```python
from build123d import *

# Parameters (mm, degrees)
SKETCH_1131_R          = 3
EXTRUDE_1145_DEPTH     = 2
EXTRUDE_1198_DEPTH     = 30
SKETCH_1301_W          = 30
SKETCH_1301_H          = 5
CUT_EXTRUDE_1405_DEPTH = 10


with BuildPart() as part:
    # Sketch 1131 → Extrude 1145 (new body)
    with BuildSketch(Plane(origin=(0, 0, 0), x_dir=(1, 0, 0), z_dir=(0, 1, 0))):
        with BuildLine():
            Line((-90, 40), (90, 40))
            ThreePointArc((90, 40), (97.071067812, 37.071067812), (100, 30))
            Line((100, 30), (100, -40))
            Line((100, -40), (-100, -40))
            Line((-100, -40), (-100, 30))
            ThreePointArc((-100, 30), (-97.071067812, 37.071067812), (-90, 40))
        make_face()
        with Locations(Location((60, -25, 0), (0, 0, 270))):
            Circle(SKETCH_1131_R, mode=Mode.SUBTRACT)
        with Locations(Location((0, -25, 0), (0, 0, 270))):
            Circle(SKETCH_1131_R, mode=Mode.SUBTRACT)
        with Locations(Location((-60, -25, 0), (0, 0, 270))):
            Circle(SKETCH_1131_R, mode=Mode.SUBTRACT)
        with BuildLine():
            Line((49, 30), (71, 30))
            ThreePointArc((71, 30), (73.828427125, 28.828427125), (75, 26))
            Line((75, 26), (75, -1))
            ThreePointArc((75, -1), (73.828427125, -3.828427125), (71, -5))
            Line((71, -5), (49, -5))
            ThreePointArc((49, -5), (46.171572875, -3.828427125), (45, -1))
            Line((45, -1), (45, 26))
            ThreePointArc((45, 26), (46.171572875, 28.828427125), (49, 30))
        make_face(mode=Mode.SUBTRACT)
        with BuildLine():
            Line((-11, 30), (11, 30))
            ThreePointArc((11, 30), (13.828427125, 28.828427125), (15, 26))
            Line((15, 26), (15, -1))
            ThreePointArc((15, -1), (13.828427125, -3.828427125), (11, -5))
            Line((11, -5), (-11, -5))
            ThreePointArc((-11, -5), (-13.828427125, -3.828427125), (-15, -1))
            Line((-15, -1), (-15, 26))
            ThreePointArc((-15, 26), (-13.828427125, 28.828427125), (-11, 30))
        make_face(mode=Mode.SUBTRACT)
        with BuildLine():
            Line((-71, 30), (-49, 30))
            ThreePointArc((-49, 30), (-46.171572875, 28.828427125), (-45, 26))
            Line((-45, 26), (-45, -1))
            ThreePointArc((-45, -1), (-46.171572875, -3.828427125), (-49, -5))
            Line((-49, -5), (-71, -5))
            ThreePointArc((-71, -5), (-73.828427125, -3.828427125), (-75, -1))
            Line((-75, -1), (-75, 26))
            ThreePointArc((-75, 26), (-73.828427125, 28.828427125), (-71, 30))
        make_face(mode=Mode.SUBTRACT)
    extrude(amount=-EXTRUDE_1145_DEPTH)

    # Sketch 1191 → Extrude 1198 (add)
    with BuildSketch(Plane(origin=(0, 0, 0), x_dir=(1, 0, 0), z_dir=(0, 1, 0))):
        with BuildLine():
            Line((-90, 40), (90, 40))
            ThreePointArc((90, 40), (97.071067812, 37.071067812), (100, 30))
            Line((100, 30), (100, -40))
            Line((100, -40), (-100, -40))
            Line((-100, -40), (-100, 30))
            ThreePointArc((-100, 30), (-97.071067812, 37.071067812), (-90, 40))
        make_face()
        with BuildLine():
            Line((-90, 35), (90, 35))
            ThreePointArc((90, 35), (93.535533906, 33.535533906), (95, 30))
            Line((95, 30), (95, -35))
            Line((95, -35), (-95, -35))
            Line((-95, -35), (-95, 30))
            ThreePointArc((-95, 30), (-93.535533906, 33.535533906), (-90, 35))
        make_face(mode=Mode.SUBTRACT)
    extrude(amount=-EXTRUDE_1198_DEPTH)

    # Sketch 1301 → Cut-Extrude 1405 (cut)
    with BuildSketch(Plane(origin=(0, -30, 0), x_dir=(1, 0, 0), z_dir=(0, 1, 0))):
        with Locations((10, 37.5)):
            Rectangle(SKETCH_1301_W, SKETCH_1301_H)
    extrude(amount=CUT_EXTRUDE_1405_DEPTH, mode=Mode.SUBTRACT)


solid = part.part
```
Source: CAD feature listing. Evaluate the final solid. Frame: model axes, mm. A direction names the side the tool comes from. Coordinates: 2 decimals unless noted, no trailing zeros. Loops run counter-clockwise (first coordinate to the right, second up) from the corner with the lowest first, then second, coordinate; pieces in that order, holes last. Notation, with made-up numbers: M -27.75,-10 L -2.75,-10 A26 cw -2.75,29 Z; hole C 15.25,55 d9. An arc over 180 degrees is marked long. Put each result on its own line as item: value. Start each with the question number.
1) Cut plane B-B on z = -16. Return the cut outline in (x, y), then the cut area to 3 significant figures.
2) Cut plane A-A on x = 0. Return the cut outline in (y, z).
3) Reachability of faces 1 (the face through (10, -20, -38)), 2 (the face through (93, -16, -34)), 3 (the face through (-46.141, -0.986, 3.797)) from +Z, -Z, +X, -X, +Y, -Y: full face, straight path, thin tool, end or side. Return the list, or none.
4) Contact query for flat-ended pins moving along their axis: pin 1 Ø5.5 at (y, z) = (-23, -37) entering from -X; pin 2 Ø9.5 at (x, z) = (0, 25) entering from +Y. Output: stop coordinate, or through.
5) Pull-direction query (Z, two-part tool) for faces 4 (the face through (-13.797, -0.986, 3.859)), 5 (the face through (-97.15, -14.79, -36.99)), 6 (the face through (73.859, -0.986, 3.797)), 7 (the face through (100, -15, 5)); classes: pulls with the +Z half, pulls with the -Z half, needs draft (parallel to the pull), parting line crosses it, or undercut.
6) Cut plane D-D on y = -7.75. Return the cut outline in (x, z), then the cut area to 3 significant figures.
7) Ray query, L1, parallel to X at y = -1.5, z = 25; L2, parallel to X at y = -20.25, z = 9.5; L3, parallel to Z at x = 52, y = -20.75. Return the intervals inside material, ascending. Write a range as from..to.
8) Cut plane C-C on x = -53. Return the cut outline in (y, z).
The answers:
1. outline: M -100,-30 L -95,-30 L -95,-2 L -75,-2 L -75,0 L -100,0 Z; M -45,-2 L -15,-2 L -15,0 L -45,0 Z; M 15,-2 L 45,-2 L 45,0 L 15,0 Z; M 75,-2 L 95,-2 L 95,-30 L 100,-30 L 100,0 L 75,0 Z
1. area: 500 mm²
2. outline: M -30,35 L -2,35 L -2,28 L 0,28 L 0,40 L -30,40 Z; M -20,-40 L 0,-40 L 0,-30 L -2,-30 L -2,-35 L -20,-35 Z; M -2,5 L 0,5 L 0,22 L -2,22 Z
3. face 1: -Z, -Y
3. face 2: -Y
3. face 3: +Y, -Y
4. pin 1: stops at x = -99.05
4. pin 2: stops at y = 0
5. face 4: undercut
5. face 5: pulls with the -Z half
5. face 6: undercut
5. face 7: needs draft
6. outline: M -100,-30 A10 ccw -90,-40 L 90,-40 A10 ccw 100,-30 L 100,40 L -100,40 Z; hole M -95,-30 A5 ccw -90,-35 L 90,-35 A5 ccw 95,-30 L 95,35 L -95,35 Z
6. area: 2,670 mm²
7. L1: x = -100..-63, -57..-3, 3..57, 63..100
7. L2: x = -100..-95, 95..100
7. L3: z = -40..-35, 35..40
8. outline: M -30,-40 L 0,-40 L 0,-30 L -2,-30 L -2,-35 L -30,-35 Z; M -30,35 L -2,35 L -2,5 L 0,5 L 0,40 L -30,40 Z
